```python
from build123d import *

# Parameters (mm, degrees)
SKETCH_1_R               = 38
EXTRUDE_1_DEPTH          = 18
CUT_EXTRUDE_1_REACH      = 58.675
SKETCH_2_R               = 1.5
CUT_EXTRUDE_2_DEPTH      = 12.5
FILLET_1_R               = 1
CUT_EXTRUDE_7_REACH      = 79.414
CUT_EXTRUDE_7_END_RADIUS = 38
SKETCH_6_W               = 20
SKETCH_6_H               = 4
CUT_EXTRUDE_8_REACH      = 58.675
SKETCH_7_R               = 1.5


with BuildPart() as part:
    # Эскиз1 → Бобышка-Вытянуть1 (new body)
    with BuildSketch(Plane.XY):
        Circle(SKETCH_1_R)
    extrude(amount=EXTRUDE_1_DEPTH)

    # Эскиз2 → Вырез-Вытянуть1 (cut, up to next)
    with BuildSketch(Plane.XY.offset(18), mode=Mode.PRIVATE) as cut_extrude_1_sk1:
        with Locations((-34, 0)):
            Circle(SKETCH_2_R)
    cut_extrude_1_tool1 = extrude(cut_extrude_1_sk1.sketch, amount=-CUT_EXTRUDE_1_REACH, mode=Mode.PRIVATE) & part.part
    # Эскиз2 → Вырез-Вытянуть1 (cut, up to next)
    with BuildSketch(Plane.XY.offset(18), mode=Mode.PRIVATE) as cut_extrude_1_sk2:
        with Locations((-17, 29.444863729)):
            Circle(SKETCH_2_R)
    cut_extrude_1_tool2 = extrude(cut_extrude_1_sk2.sketch, amount=-CUT_EXTRUDE_1_REACH, mode=Mode.PRIVATE) & part.part
    # Эскиз2 → Вырез-Вытянуть1 (cut, up to next)
    with BuildSketch(Plane.XY.offset(18), mode=Mode.PRIVATE) as cut_extrude_1_sk3:
        with Locations((17, 29.444863729)):
            Circle(SKETCH_2_R)
    cut_extrude_1_tool3 = extrude(cut_extrude_1_sk3.sketch, amount=-CUT_EXTRUDE_1_REACH, mode=Mode.PRIVATE) & part.part
    # Эскиз2 → Вырез-Вытянуть1 (cut, up to next)
    with BuildSketch(Plane.XY.offset(18), mode=Mode.PRIVATE) as cut_extrude_1_sk4:
        with Locations((34, 0)):
            Circle(SKETCH_2_R)
    cut_extrude_1_tool4 = extrude(cut_extrude_1_sk4.sketch, amount=-CUT_EXTRUDE_1_REACH, mode=Mode.PRIVATE) & part.part
    # Эскиз2 → Вырез-Вытянуть1 (cut, up to next)
    with BuildSketch(Plane.XY.offset(18), mode=Mode.PRIVATE) as cut_extrude_1_sk5:
        with Locations((17, -29.444863729)):
            Circle(SKETCH_2_R)
    cut_extrude_1_tool5 = extrude(cut_extrude_1_sk5.sketch, amount=-CUT_EXTRUDE_1_REACH, mode=Mode.PRIVATE) & part.part
    # Эскиз2 → Вырез-Вытянуть1 (cut, up to next)
    with BuildSketch(Plane.XY.offset(18), mode=Mode.PRIVATE) as cut_extrude_1_sk6:
        with Locations((-17, -29.444863729)):
            Circle(SKETCH_2_R)
    cut_extrude_1_tool6 = extrude(cut_extrude_1_sk6.sketch, amount=-CUT_EXTRUDE_1_REACH, mode=Mode.PRIVATE) & part.part
    add(cut_extrude_1_tool1.solids().sort_by_distance((-34, 0, 18))[0], mode=Mode.SUBTRACT)
    add(cut_extrude_1_tool2.solids().sort_by_distance((-17, 29.444864, 18))[0], mode=Mode.SUBTRACT)
    add(cut_extrude_1_tool3.solids().sort_by_distance((17, 29.444864, 18))[0], mode=Mode.SUBTRACT)
    add(cut_extrude_1_tool4.solids().sort_by_distance((34, 0, 18))[0], mode=Mode.SUBTRACT)
    add(cut_extrude_1_tool5.solids().sort_by_distance((17, -29.444864, 18))[0], mode=Mode.SUBTRACT)
    add(cut_extrude_1_tool6.solids().sort_by_distance((-17, -29.444864, 18))[0], mode=Mode.SUBTRACT)

    # Эскиз3 → Вырез-Вытянуть2 (cut)
    with BuildSketch(Plane(origin=(0, 0, 0), x_dir=(-1, 0, 0), z_dir=(0, 0, -1))):
        with BuildLine():
            Line((-13.076696831, -27), (13.076696831, -27))
            ThreePointArc((13.076696831, -27), (0, 30), (-13.076696831, -27))
        make_face()
    extrude(amount=-CUT_EXTRUDE_2_DEPTH, mode=Mode.SUBTRACT)

    # Скругление1
    fillet_1_edges = [part.edges().sort_by_distance(p)[0] for p in [
        (-38, 0, 18),
    ]]
    fillet(fillet_1_edges, radius=FILLET_1_R)

    # Вырез-Вытянуть7: up to this cylinder (the profile starts inside it)
    cut_extrude_7_end = Plane(origin=(0, 0, 10.5), z_dir=(0, 0, -1)) * Cylinder(CUT_EXTRUDE_7_END_RADIUS, 235.828, mode=Mode.PRIVATE)
    # Эскиз6 → Вырез-Вытянуть7 (cut, up to the surface)
    with BuildSketch(Plane(origin=(0, -27, 0), x_dir=(1, 0, 0), z_dir=(0, 1, 0)), mode=Mode.PRIVATE) as cut_extrude_7_sk1:
        with Locations((0, -10.5)):
            Rectangle(SKETCH_6_W, SKETCH_6_H)
    cut_extrude_7_tool1 = extrude(cut_extrude_7_sk1.sketch, amount=-CUT_EXTRUDE_7_REACH, mode=Mode.PRIVATE) & cut_extrude_7_end
    add(cut_extrude_7_tool1.solids().sort_by_distance((0, -27, 10.5))[0], mode=Mode.SUBTRACT)

    # Эскиз7 → Вырез-Вытянуть8 (cut, up to next)
    with BuildSketch(Plane.XY.offset(18), mode=Mode.PRIVATE) as cut_extrude_8_sk1:
        with Locations((-18, 0)):
            Circle(SKETCH_7_R)
    cut_extrude_8_tool1 = extrude(cut_extrude_8_sk1.sketch, amount=-CUT_EXTRUDE_8_REACH, mode=Mode.PRIVATE) & part.part
    # Эскиз7 → Вырез-Вытянуть8 (cut, up to next)
    with BuildSketch(Plane.XY.offset(18), mode=Mode.PRIVATE) as cut_extrude_8_sk2:
        with Locations((-9, 15.588457268)):
            Circle(SKETCH_7_R)
    cut_extrude_8_tool2 = extrude(cut_extrude_8_sk2.sketch, amount=-CUT_EXTRUDE_8_REACH, mode=Mode.PRIVATE) & part.part
    # Эскиз7 → Вырез-Вытянуть8 (cut, up to next)
    with BuildSketch(Plane.XY.offset(18), mode=Mode.PRIVATE) as cut_extrude_8_sk3:
        with Locations((9, 15.588457268)):
            Circle(SKETCH_7_R)
    cut_extrude_8_tool3 = extrude(cut_extrude_8_sk3.sketch, amount=-CUT_EXTRUDE_8_REACH, mode=Mode.PRIVATE) & part.part
    # Эскиз7 → Вырез-Вытянуть8 (cut, up to next)
    with BuildSketch(Plane.XY.offset(18), mode=Mode.PRIVATE) as cut_extrude_8_sk4:
        with Locations((18, 0)):
            Circle(SKETCH_7_R)
    cut_extrude_8_tool4 = extrude(cut_extrude_8_sk4.sketch, amount=-CUT_EXTRUDE_8_REACH, mode=Mode.PRIVATE) & part.part
    # Эскиз7 → Вырез-Вытянуть8 (cut, up to next)
    with BuildSketch(Plane.XY.offset(18), mode=Mode.PRIVATE) as cut_extrude_8_sk5:
        with Locations((9, -15.588457268)):
            Circle(SKETCH_7_R)
    cut_extrude_8_tool5 = extrude(cut_extrude_8_sk5.sketch, amount=-CUT_EXTRUDE_8_REACH, mode=Mode.PRIVATE) & part.part
    # Эскиз7 → Вырез-Вытянуть8 (cut, up to next)
    with BuildSketch(Plane.XY.offset(18), mode=Mode.PRIVATE) as cut_extrude_8_sk6:
        with Locations((-9, -15.588457268)):
            Circle(SKETCH_7_R)
    cut_extrude_8_tool6 = extrude(cut_extrude_8_sk6.sketch, amount=-CUT_EXTRUDE_8_REACH, mode=Mode.PRIVATE) & part.part
    add(cut_extrude_8_tool1.solids().sort_by_distance((-18, 0, 18))[0], mode=Mode.SUBTRACT)
    add(cut_extrude_8_tool2.solids().sort_by_distance((-9, 15.588457, 18))[0], mode=Mode.SUBTRACT)
    add(cut_extrude_8_tool3.solids().sort_by_distance((9, 15.588457, 18))[0], mode=Mode.SUBTRACT)
    add(cut_extrude_8_tool4.solids().sort_by_distance((18, 0, 18))[0], mode=Mode.SUBTRACT)
    add(cut_extrude_8_tool5.solids().sort_by_distance((9, -15.588457, 18))[0], mode=Mode.SUBTRACT)
    add(cut_extrude_8_tool6.solids().sort_by_distance((-9, -15.588457, 18))[0], mode=Mode.SUBTRACT)


solid = part.part
```
Geometry: final body of the model. Coordinates: model frame, mm. A direction names the side the tool comes from. Round coordinates to 2 decimals unless told otherwise and drop trailing zeros. Write each loop counter-clockwise with the first axis right and the second up, starting at its lowest first coordinate (ties: lowest second). Pieces come first, ordered by that corner, then holes. Notation, with made-up numbers: M 22,74.5 L 79,74.5 A28 cw 79,108.5 Z; hole C 79.25,78.5 d8. An arc over 180 degrees is marked long. Answer in a Markdown table with one row per item. Add a question column.
(1) Contact query for flat-ended pins moving along their axis: pin 1 (4.5 mm diameter, centred on y = -30.5, z = 10, fed in from -X); pin 2 (2.5 mm diameter, centred on x = -9, y = 15.59, fed in from +Z); pin 3 (8 mm diameter, centred on x = -8, z = 5.5, fed in from +Y); pin 4 (4 mm diameter, centred on x = -18, y = 0, fed in from -Z). Output: stop coordinate, or through.
(2) Reachability of faces 1 (the face through (10, -32, 11)), 2 (the face through (-19.5, 0.07, 15.29)), 3 (the face through (-1.13, 29.98, 6.16)) from +Z, -Z, +X, -X, +Y, -Y: full face, straight path, thin tool, end or side. Return the list, or none.
(3) Ray query, L1, parallel to Z at x = 2.5, y = -34; L2, parallel to X at y = 1, z = 8.25; L3, parallel to Y at x = 9, z = 16.3. Return the intervals inside material, ascending.
(4) Draft query along Z for faces 4 (the face through (0, -32, 8.5)), 5 (the face through (-9.325, 14.124, 15.288)), 6 (the face through (0, -28, 0)). Return one class per face: pulls with the +Z half, pulls with the -Z half, needs draft (parallel to the pull), parting line crosses it, or undercut.
(5) Cut plane B-B, the plane z = 2. Return the cut outline in (x, y).
(6) Cut plane C-C, the plane x = -9. Give the number of separate pieces and of enclosed holes in the cut face, then the cut area to 3 significant figures.
(7) Cut plane A-A, the plane z = 11.25. Return the cut outline in (x, y), then the cut area to 3 significant figures.
Established:
| question | item | result |
|---|---|---|
| 1 | pin 1 | x = -25.42 |
| 1 | pin 2 | through |
| 1 | pin 3 | y = 37.79 |
| 1 | pin 4 | z = 12.5 |
| 2 | face 1 | -Y |
| 2 | face 2 | +Z, -Z |
| 2 | face 3 | -Z |
| 3 | L1 | 0 to 8.5, 12.5 to 18 |
| 3 | L2 | -37.99 to -35.12, -32.88 to -29.98, 29.98 to 32.88, 35.12 to 37.99 |
| 3 | L3 | -36.92 to -17.09, -14.09 to 14.09, 17.09 to 36.92 |
| 4 | face 4 | undercut |
| 4 | face 5 | needs draft |
| 4 | face 6 | pulls with the -Z half |
| 5 | outline | C 0,0 d76; hole C -34,0 d3; hole C -17,-29.44 d3; hole C -17,29.44 d3; hole M -13.08,-27 L 13.08,-27 A30 ccw long Z; hole C 17,-29.44 d3; hole C 17,29.44 d3; hole C 34,0 d3 |
| 6 | separate pieces | 4 |
| 6 | enclosed holes | 0 |
| 6 | area | 561 mm² |
| 7 | outline | M -13.08,-27 A30 cw long 13.08,-27 L 10,-27 L 10,-36.66 A38 ccw long -10,-36.66 L -10,-27 Z; hole C -34,0 d3; hole C -17,-29.44 d3; hole C -17,29.44 d3; hole C 17,-29.44 d3; hole C 17,29.44 d3; hole C 34,0 d3 |
| 7 | area | 1,510 mm² |
